from build123d import *

# Parameters (mm, degrees)
SKETCH1_W           = 63.5
SKETCH1_H           = 63.5
BOSS_EXTRUDE1_DEPTH = 12.7
SKETCH2_W           = 63.5
SKETCH2_H           = 3.175
CUT_EXTRUDE1_DEPTH  = 3.175
SKETCH3_W           = 6.35
SKETCH3_H           = 12.7
BOSS_EXTRUDE2_DEPTH = 12.7
SKETCH4_R           = 3.175
CUT_EXTRUDE2_DEPTH  = 64.5


with BuildPart() as part:
    # Sketch1 → Boss-Extrude1 (new body)
    with BuildSketch(Plane(origin=(0, 0, 0), x_dir=(1, 0, 0), z_dir=(0, 1, 0))):
        Rectangle(SKETCH1_W, SKETCH1_H)
        with BuildLine():
            Line((-23.540128061, -14.559871939), (14.559871939, 23.540128061))
            ThreePointArc((14.559871939, 23.540128061), (23.540128061, 23.540128061), (23.540128061, 14.559871939))
            Line((23.540128061, 14.559871939), (-14.559871939, -23.540128061))
            ThreePointArc((-14.559871939, -23.540128061), (-23.540128061, -23.540128061), (-23.540128061, -14.559871939))
        make_face(mode=Mode.SUBTRACT)
    extrude(amount=BOSS_EXTRUDE1_DEPTH)

    # Sketch2 → Cut-Extrude1 (cut)
    with BuildSketch(Plane.XY.offset(31.75)):
        with Locations((0, 6.35)):
            Rectangle(SKETCH2_W, SKETCH2_H)
    cut_extrude1 = extrude(amount=-CUT_EXTRUDE1_DEPTH, mode=Mode.SUBTRACT)

    # Mirror1: Cut-Extrude1 across plane
    add(cut_extrude1.mirror(Plane.XY), mode=Mode.SUBTRACT)

    # Sketch3 → Boss-Extrude2 (add)
    with BuildSketch(Plane(origin=(0, 12.7, 0), x_dir=(1, 0, 0), z_dir=(0, 1, 0))):
        with Locations((-28.575, 0)):
            Rectangle(SKETCH3_W, SKETCH3_H)
    extrude(amount=BOSS_EXTRUDE2_DEPTH)

    # Sketch4 → Cut-Extrude2 (cut, through all)
    with BuildSketch(Plane.ZY.offset(31.75)):
        with Locations((0, 19.05)):
            Circle(SKETCH4_R)
    extrude(amount=-CUT_EXTRUDE2_DEPTH, mode=Mode.SUBTRACT)


solid = part.part
The listing builds one solid part. Answer for the finished solid, in the listing's coordinates (mm). A direction names the side the tool comes from. Coordinates: 2 decimals unless noted, no trailing zeros. Loops run counter-clockwise (first coordinate to the right, second up) from the corner with the lowest first, then second, coordinate; pieces in that order, holes last.
1) Find section A-A on y = 2.5. Write down the section's boundary in (x, z), then the cut area to 3 significant figures.
2) Flat-ended cylindrical pins translate along their axes: pin 1 Ø10 at (y, z) = (21.5, 22) entering from -X; pin 2 Ø1 at (x, y) = (10.5, 7) entering from +Z (3 decimals); pin 3 Ø1.6 at (x, z) = (-14, 29.5) entering from +Y; pin 4 Ø7 at (x, y) = (-29.5, 21.5) entering from +Z. Find the tip coordinate at first contact, or state that the pin passes through.
3) Determine the mould class of faces 1 (the face through (4.76, 6.26, 4.22)), 2 (the face through (-29, 19, 6.35)), 3 (the face through (0, 10, -31.75)), 4 (the face through (0, 4.762, 30)) for opening direction Z: pulls with the +Z half, pulls with the -Z half, needs draft (parallel to the pull), parting line crosses it, or undercut.
4) A tool of negligible diameter and unlimited length cuts with its end or side. For faces 5 (the face through (0, 6, -28.575)), 6 (the face through (0, 6, 28.575)), 7 (the face through (0, 2, -31.75)), 8 (the face through (-25.4, 16, 2)), 9 (the face through (-29, 25.4, 0)), from which of +Z, -Z, +X, -X, +Y, -Y can it reach the whole face along a straight path? Write none if from no direction.
5) Find the intervals of material crossed by L1, parallel to Y at x = -28, z = 0 (3 decimals); L2, parallel to Y at x = -24.5, z = -7.5; L3, parallel to Y at x = 6, z = -29, in increasing order.
6) Find section B-B on z = 24.5. Write down the section's boundary in (x, y).
7) Find section D-D on y = 19.05. Write down the section's boundary in (x, z) (3 decimals).
Values:
1. outline: (-31.75, -31.75) - (31.75, -31.75) - (31.75, 31.75) - (-31.75, 31.75) - close; hole (-23.54, 14.56) - (14.56, -23.54) arc R6.35 ccw to (23.54, -14.56) - (-14.56, 23.54) arc R6.35 ccw to start
1. area: 3,220 mm2
2. pin 1: passes through
2. pin 2: stops at z = 28.575
2. pin 3: stops at y = 12.7
2. pin 4: stops at z = 6.35
3. face 1: undercut
3. face 2: pulls with the +Z half
3. face 3: pulls with the -Z half
3. face 4: needs draft
4. face 5: -Z, +X, -X
4. face 6: +Z, +X, -X
4. face 7: -Z, +X, -X, +Y, -Y
4. face 8: +Z, -Z, +X, +Y
4. face 9: +Z, -Z, +X, -X, +Y
5. L1: y = 0 to 15.875, 22.225 to 25.4
5. L2: y = 0 to 12.7
5. L3: y = 0 to 4.76, 7.94 to 12.7
6. outline: (-31.75, 0) - (-22.31, 0) - (-22.31, 12.7) - (-31.75, 12.7) - close; (-15.79, 0) - (31.75, 0) - (31.75, 12.7) - (-15.79, 12.7) - close
7. outline: (-31.75, -6.35) - (-25.4, -6.35) - (-25.4, -3.175) - (-31.75, -3.175) - close; (-31.75, 3.175) - (-25.4, 3.175) - (-25.4, 6.35) - (-31.75, 6.35) - close
